Geometry: final body of the model. Coordinates: model frame, mm. Face numbers are marked on the shaded views. A direction names the side the tool comes from. Round coordinates to 2 decimals unless told otherwise and drop trailing zeros. Order: outer loops, then holes, each group sorted by start corner. A loop starts at its lowest first (then second) coordinate and runs counter-clockwise, first axis right, second up. Notation, with made-up numbers: M 33,11 L 54,11 A23 ccw 54,21 Z; hole C 82,51.5 d10. An arc over 180 degrees is marked long. Return JSON: item names as keys, results as strings. Group by question number.
Q1. Cut plane A-A on y = 2.5. Output: boundary loops of the cut face in (x, z), and give its area (3 significant figures).
Q2. Ray query, probe 1 along X at (y, z) = (6, -0.75); probe 2 along Z at (x, y) = (10, 0.75); probe 3 along X at (y, z) = (3.5, 0.5). Return the intervals inside material, ascending.
Q3. Cut plane D-D on z = -6. Output: boundary loops of the cut face in (x, y), and give its area (3 significant figures).
Q4. Cut plane B-B on z = -2.75. Output: boundary loops of the cut face in (x, y).
Q5. Cut plane C-C on x = -17. Output: boundary loops of the cut face in (y, z).
Q6. Contact query for flat-ended pins moving along their axis: pin 1 (1.5 mm diameter, centred on x = -0.5, y = 3, fed in from +Z); pin 2 (8 mm diameter, centred on x = -19, z = 2.5, fed in from +Y); pin 3 (4 mm diameter, centred on y = 5.5, z = -4.5, fed in from -X); pin 4 (3 mm diameter, centred on x = -28, z = 5.5, fed in from -Y). Output: stop coordinate, or through.
Q7. Access query for the marked faces 1, 2 and 3. Directions: +Z, -Z, +X, -X, +Y, -Y. A direction counts if a zero-diameter tool reaches every point of the face in a straight line with its end or side. Return the directions, or none.
```python
from build123d import *

# Parameters (mm, degrees)
BOSS_EXTRUDE1_DEPTH = 7.5
FILLET1_R           = 30
FILLET2_R           = 30


with BuildPart() as part:
    # Sketch1 → Boss-Extrude1 (new body)
    with BuildSketch(Plane(origin=(0, 0, 0), x_dir=(1, 0, 0), z_dir=(0, 1, 0))):
        with BuildLine():
            ThreePointArc((-58.191489362, -2.446808511), (-61.191489362, 0.553191489), (-58.191489362, 3.553191489))
            Line((-58.191489362, 3.553191489), (-51.317625819, 3.553191489))
            ThreePointArc((-51.317625819, 3.553191489), (-65.691489362, 0.553191489), (-51.317625819, -2.446808511))
            Line((-51.317625819, -2.446808511), (-58.191489362, -2.446808511))
        make_face()
        with BuildLine():
            Line((-51.317625819, 3.553191489), (-58.191489362, 3.553191489))
            ThreePointArc((-58.191489362, 3.553191489), (-56.070169018, 2.674511833), (-55.191489362, 0.553191489))
            ThreePointArc((-55.191489362, 0.553191489), (-56.070169018, -1.568128854), (-58.191489362, -2.446808511))
            Line((-58.191489362, -2.446808511), (-51.317625819, -2.446808511))
            ThreePointArc((-51.317625819, -2.446808511), (-50.849692015, -0.979130838), (-50.691489362, 0.553191489))
            ThreePointArc((-50.691489362, 0.553191489), (-50.849692015, 2.085513817), (-51.317625819, 3.553191489))
        make_face()
        with BuildLine():
            Line((16.808510638, 3.553191489), (-51.317625819, 3.553191489))
            ThreePointArc((-51.317625819, 3.553191489), (-50.849692015, 2.085513817), (-50.691489362, 0.553191489))
            ThreePointArc((-50.691489362, 0.553191489), (-50.849692015, -0.979130838), (-51.317625819, -2.446808511))
            Line((-51.317625819, -2.446808511), (16.808510638, -2.446808511))
            Line((16.808510638, -2.446808511), (16.808510638, 3.553191489))
        make_face()
    extrude(amount=BOSS_EXTRUDE1_DEPTH)

    # Fillet1
    fillet1_edges = [part.edges().sort_by_distance(p)[0] for p in [
        (-51.317625819, 3.75, 2.446808511),
    ]]
    fillet(fillet1_edges, radius=FILLET1_R)

    # Fillet2
    fillet2_edges = [part.edges().sort_by_distance(p)[0] for p in [
        (-51.317625819, 3.75, -3.553191489),
    ]]
    fillet(fillet2_edges, radius=FILLET2_R)


solid = part.part
```
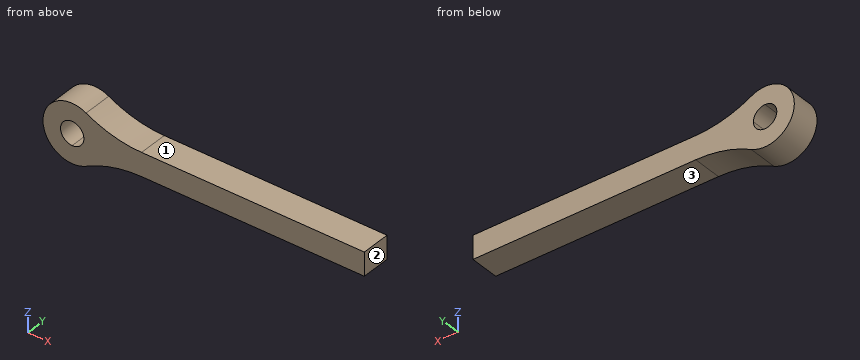
Result sheet:
{
 "1": {"outline": "M -54.63,-7.15 A30 cw -40.38,-3.55 L 16.81,-3.55 L 16.81,2.45 L -40.38,2.45 A30 cw -54.63,6.05 A7.5 ccw long Z; hole C -58.19,-0.55 d6", "area": "573 mm²"},
 "2": {"probe 1": "x = -65.69 to -61.19, -55.2 to 16.81", "probe 2": "z = -3.55 to 2.45", "probe 3": "x = -65.62 to -61, -55.38 to 16.81"},
 "3": {"outline": "M -63.35,0 L -52.25,0 L -52.25,7.5 L -63.35,7.5 Z", "area": "83.3 mm²"},
 "4": {"outline": "M -65.36,0 L -60.23,0 L -60.23,7.5 L -65.36,7.5 Z; M -56.15,0 L 16.81,0 L 16.81,7.5 L -56.15,7.5 Z"},
 "5": {"outline": "M 0,-3.55 L 7.5,-3.55 L 7.5,2.45 L 0,2.45 Z"},
 "6": {"pin 1": "stops at z = 2.45", "pin 2": "stops at y = 7.5", "pin 3": "stops at x = -65.43", "pin 4": "passes through"},
 "7": {"face 1": "+Z, +X, +Y, -Y", "face 2": "+Z, -Z, +X, +Y, -Y", "face 3": "-Z, +X, +Y, -Y"}
}
